from build123d import *

# Parameters (mm, degrees)
F0_R     = 23.8741589036
F1_DEPTH = 25.4
F2_R     = 17.78
F4_D     = 6.35
F4_DEPTH = 6.35
F4_TIP   = 1.9077324654
F5_R     = 1.27


with BuildPart() as f1:
    # F0 (on Right) → F1 (new body)
    with BuildSketch(Plane.YZ):
        with Locations((0, 17.5948925316)):
            Circle(F0_R)
    extrude(amount=-F1_DEPTH)

    # F2
    f2_edges = [f1.edges().sort_by_distance(p)[0] for p in [
        (0, -23.874159, 17.594893),
    ]]
    fillet(f2_edges, radius=F2_R)

    # F4
    with Locations(Plane(origin=(-25.4, 0, 0), x_dir=(0, -1, 0), z_dir=(-1, 0, 0))):
        with Locations((0, 17.5948925316)):
            Hole(F4_D / 2, depth=F4_DEPTH)
            with Locations((0, 0, -(F4_DEPTH + F4_TIP / 2))):  # 118° drill point
                Cone(0, F4_D / 2, F4_TIP, mode=Mode.SUBTRACT)

    # F5
    f5_edges = [f1.edges().sort_by_distance(p)[0] for p in [
        (-25.4, -23.874159, 17.594893),
    ]]
    fillet(f5_edges, radius=F5_R)


solid = f1.part
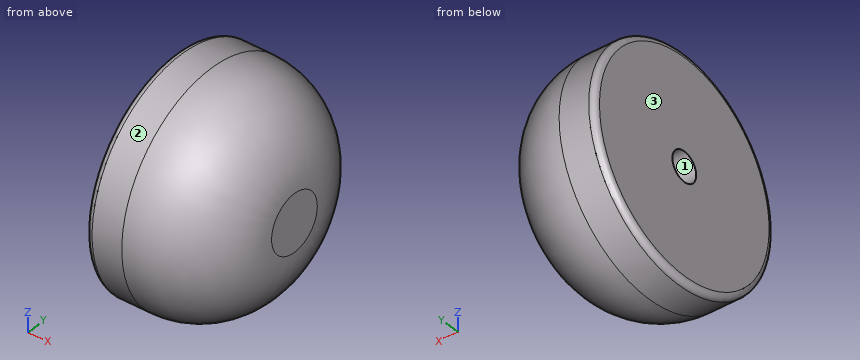
Verification items for the finished model (mm, model axes). Face numbers are marked on the shaded views. Coordinates: 2 decimals unless noted, no trailing zeros. Write each loop counter-clockwise with the first axis right and the second up, starting at its lowest first coordinate (ties: lowest second). Pieces come first, ordered by that corner, then holes. Notation, with made-up numbers: M -1.75,36 L 3.25,36 A21 cw 3.25,75 Z; hole C 89,49 d1. An arc over 180 degrees is marked long. Use a Markdown table: item, result.
Q1. Go/stop test with flat-tipped pins: P1, Ø8, axis at x = -5, y = 14, coming from the -Z side; P2, Ø6, axis at x = -11.5, z = 6, coming from the -Y side; P3, Ø2, axis at x = -17, y = 16, coming from the -Z side. Record where each tip stops, or that it passes through.
Reply:
| item | result |
|---|---|
| P1 | stops at z = 0 |
| P2 | stops at y = -21.41 |
| P3 | stops at z = -0.96 |
Q2. Thickness scan on line 1 (Z direction, x = -23.5, y = 0); line 2 (X direction, y = 9.5, z = -2.5); line 3 (Z direction, x = -24, y = 2). Record the ranges inside material, lowest first.
Reply:
| item | result |
|---|---|
| line 1 | z = -6.28 to 14.42, 20.77 to 41.47 |
| line 2 | x = -25.4 to -10.31 |
| line 3 | z = -6.2 to 15.13, 20.06 to 41.39 |
Q3. Sectioned sample at A-A, the plane x = -22. Record the boundary of the cut face in (y, z) (3 decimals).
Reply:
| item | result |
|---|---|
| outline | C 0,17.595 d47.748; hole C 0,17.595 d6.35 |
Q4. Draft check along Y on the marked faces 1, 2 and 3. Enter one of: +Y half, -Y half, draft (parallel to the pull), parting line (faces both ways), or undercut.
Reply:
| item | result |
|---|---|
| face 1 | undercut |
| face 2 | parting line |
| face 3 | draft |
